Verification items for the finished model (mm, model axes). A direction names the side the tool comes from. Round coordinates to 2 decimals unless told otherwise and drop trailing zeros. Loops run counter-clockwise (first coordinate to the right, second up) from the corner with the lowest first, then second, coordinate; pieces in that order, holes last. Notation, with made-up numbers: (77.5, 61) -> (128.5, 61) arc R19 cw to (128.5, 90) -> close; hole circle Ø10 at (83, 68). An arc over 180 degrees is marked (long way). Write item = value, one per line.
```python
from build123d import *

# Parameters (mm, degrees)
SKETCH_1_W          = 90
SKETCH_1_H          = 20
SKETCH_1_R          = 1.75
EXTRUDE_1_DEPTH     = 4
SKETCH_2_W          = 4
SKETCH_2_H          = 20
EXTRUDE_2_DEPTH     = 32
SKETCH_3_W          = 60
SKETCH_3_H          = 20
SKETCH_3_R          = 8.1
EXTRUDE_3_DEPTH     = 4
FILLET_1_R          = 5
FILLET_2_R          = 3
SKETCH_4_W          = 19
SKETCH_4_H          = 20
CUT_EXTRUDE_1_DEPTH = 1
SKETCH_5_R          = 3.1
CUT_EXTRUDE_2_DEPTH = 10
SKETCH_6_W          = 13.6
SKETCH_6_H          = 7.5
CUT_EXTRUDE_3_DEPTH = 1
SKETCH_7_R          = 5.25
CUT_EXTRUDE_4_DEPTH = 1


with BuildPart() as part:
    # 草图1 → 凸台-拉伸1 (new body)
    with BuildSketch(Plane(origin=(0, 0, 0), x_dir=(1, 0, 0), z_dir=(0, 1, 0))):
        with Locations((45, 10)):
            Rectangle(SKETCH_1_W, SKETCH_1_H)
        with Locations(Location((85, 10, 0), (0, 0, 270))):
            Circle(SKETCH_1_R, mode=Mode.SUBTRACT)
        with Locations(Location((5, 10, 0), (0, 0, 90))):
            Circle(SKETCH_1_R, mode=Mode.SUBTRACT)
    extrude(amount=EXTRUDE_1_DEPTH)

    # 草图2 → 凸台-拉伸2 (add)
    with BuildSketch(Plane(origin=(0, 4, 0), x_dir=(1, 0, 0), z_dir=(0, 1, 0))):
        with Locations((17, 10)):
            Rectangle(SKETCH_2_W, SKETCH_2_H)
        with Locations((73, 10)):
            Rectangle(SKETCH_2_W, SKETCH_2_H)
    extrude(amount=EXTRUDE_2_DEPTH)

    # 草图3 → 凸台-拉伸3 (add)
    with BuildSketch(Plane(origin=(0, 36, 0), x_dir=(1, 0, 0), z_dir=(0, 1, 0))):
        with Locations((45, 10)):
            Rectangle(SKETCH_3_W, SKETCH_3_H)
        with Locations(Location((58, 10, 0), (0, 0, 270))):
            Circle(SKETCH_3_R, mode=Mode.SUBTRACT)
    extrude(amount=EXTRUDE_3_DEPTH)

    # 圆角1
    fillet_1_edges = [part.edges().sort_by_distance(p)[0] for p in [
        (15, 4, -10),
        (19, 4, -10),
        (75, 4, -10),
        (71, 4, -10),
    ]]
    fillet(fillet_1_edges, radius=FILLET_1_R)

    # 圆角2
    fillet_2_edges = [part.edges().sort_by_distance(p)[0] for p in [
        (19, 36, -10),
        (71, 36, -10),
    ]]
    fillet(fillet_2_edges, radius=FILLET_2_R)

    # 草图4 → 切除-拉伸1 (cut)
    with BuildSketch(Plane(origin=(0, 40, 0), x_dir=(1, 0, 0), z_dir=(0, 1, 0))):
        with Locations((58, 10)):
            Rectangle(SKETCH_4_W, SKETCH_4_H)
    extrude(amount=-CUT_EXTRUDE_1_DEPTH, mode=Mode.SUBTRACT)

    # 草图5 → 切除-拉伸2 (cut)
    with BuildSketch(Plane(origin=(0, 40, 0), x_dir=(1, 0, 0), z_dir=(0, 1, 0))):
        with Locations(Location((33.5, 10, 0), (0, 0, 270))):
            Circle(SKETCH_5_R)
    extrude(amount=-CUT_EXTRUDE_2_DEPTH, mode=Mode.SUBTRACT)

    # 草图6 → 切除-拉伸3 (cut)
    with BuildSketch(Plane.XZ.offset(-36)):
        with Locations((33.5, -10)):
            Rectangle(SKETCH_6_W, SKETCH_6_H)
    extrude(amount=-CUT_EXTRUDE_3_DEPTH, mode=Mode.SUBTRACT)

    # 草图7 → 切除-拉伸4 (cut)
    with BuildSketch(Plane(origin=(0, 40, 0), x_dir=(1, 0, 0), z_dir=(0, 1, 0))):
        with Locations(Location((33.5, 10, 0), (0, 0, 270))):
            Circle(SKETCH_7_R)
    extrude(amount=-CUT_EXTRUDE_4_DEPTH, mode=Mode.SUBTRACT)


solid = part.part
```
(1) Go/stop test with flat-tipped pins: pin 1 Ø10 at (y, z) = (10, -17.5) entering from -X; pin 2 Ø7 at (x, z) = (33.5, -10) entering from -Y; pin 3 Ø0.8 at (y, z) = (36.5, -11) entering from -X; pin 4 Ø11 at (x, z) = (87.5, -11.5) entering from +Y. Record where each tip stops, or that it passes through.
Filled sheet:
pin_1 = 13
pin_2 = 0
pin_3 = 15
pin_4 = 4
(2) Sectioned sample at B-B, the plane y = 26. Record the cut outline in (x, z).
Filled sheet:
outline = (15, -20) -> (19, -20) -> (19, 0) -> (15, 0) -> close; (71, -20) -> (75, -20) -> (75, 0) -> (71, 0) -> close
(3) Draft check along Y on faces 1 (the face through (70.1, 35.14, -10.14)), 2 (the face through (21, 5, -10)), 3 (the face through (37.93, 39.51, -7.18)), 4 (the face through (44, 0, -10)). Enter one of: released by +Y, released by -Y, zero draft, split by the parting line, or undercut.
Filled sheet:
face_1 = undercut
face_2 = undercut
face_3 = zero draft
face_4 = released by -Y
(4) Sectioned sample at C-C, the plane x = 58. Record the cut outline in (y, z).
Filled sheet:
outline = (0, -20) -> (4, -20) -> (4, 0) -> (0, 0) -> close; (36, -20) -> (39, -20) -> (39, -18.1) -> (36, -18.1) -> close; (36, -1.9) -> (39, -1.9) -> (39, 0) -> (36, 0) -> close
(5) Material ranges on probe 1 along X at (y, z) = (37.6, -10); probe 2 along X at (y, z) = (39.7, -10); probe 3 along Y at (x, z) = (48, -3.5), recorded low to high. Write a range as from..to.
Filled sheet:
probe_1 = 15..30.4, 36.6..49.9, 66.1..75
probe_2 = 15..28.25, 38.75..48.5, 67.5..75
probe_3 = 0..4, 36..40
(6) Sectioned sample at D-D, the plane z = -10. Count the separate pieces of the cut face and the enclosed holes in it, and give its area (3 significant figures).
Filled sheet:
separate_pieces = 4
enclosed_holes = 0
area = 749 mm2
(7) Set-up check for faces 5 (the face through (36.574, 38.014, -10.404)), 6 (the face through (7, 4, -10)), 7 (the face through (71, 21, -10)): record each of +Z, -Z, +X, -X, +Y, -Y from which the full face is reachable in a straight line by a thin tool's end or side.
Filled sheet:
face_5 = +Y
face_6 = +Z, -Z, -X, +Y
face_7 = +Z, -Z
(8) Sectioned sample at A-A, the plane x = 85. Record the cut outline in (y, z).
Filled sheet:
outline = (0, -20) -> (4, -20) -> (4, -11.75) -> (0, -11.75) -> close; (0, -8.25) -> (4, -8.25) -> (4, 0) -> (0, 0) -> close
